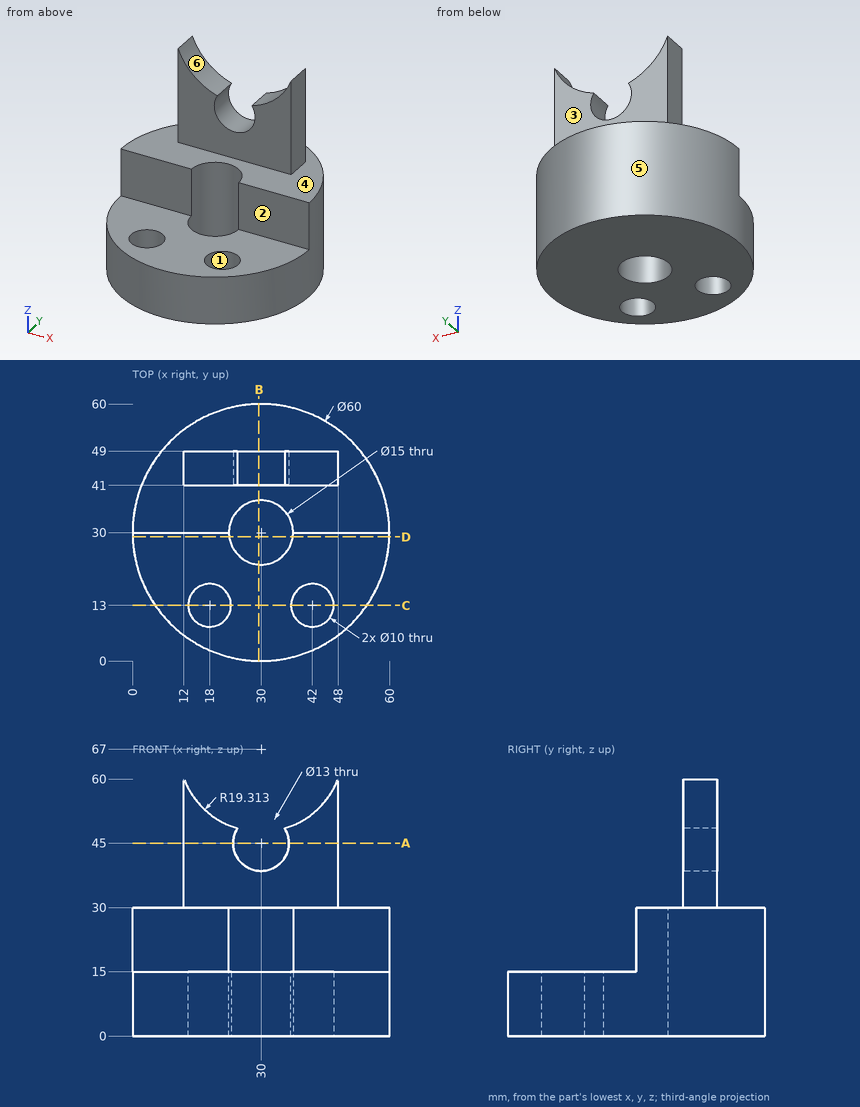
Source: three-view drawing plus pictorial views. Frame: mm from the lowest corner of the part. A direction names the side the tool comes from. Coordinates: 2 decimals unless noted, no trailing zeros. Order: outer loops, then holes, each group sorted by start corner. A loop starts at its lowest first (then second) coordinate and runs counter-clockwise, first axis right, second up. Notation, with made-up numbers: M -16.75,69 L 42.25,69 A14 ccw 42.25,84 Z; hole C -22,58.5 d11. An arc over 180 degrees is marked long. Write each question's results on one line, items separated by ' | '. Start each with the question number.
1. Section B-B, the plane x = 29.5. Return the cut outline in (y, z), then the cut area to 3 significant figures.
2. Section C-C, the plane y = 13. Return the cut outline in (x, z).
3. Reachability of the marked faces 1, 2 and 3 from +Z, -Z, +X, -X, +Y, -Y: full face, straight path, thin tool, end or side. Return the list, or none.
4. Pin query (flat end, axial travel): pin 1 (9 mm diameter, centred on x = 30, y = 30, fed in from -Z); pin 2 (1.5 mm diameter, centred on x = 26.5, y = 36.5, fed in from +Z); pin 3 (7.5 mm diameter, centred on x = 50.5, z = 24.5, fed in from -Y); pin 4 (10 mm diameter, centred on y = 36.5, z = 49, fed in from -X). Return the tip coordinate at first contact, or that it passes through.
5. Draft query along X for the marked faces 4, 5 and 6. Return one class per face: +X half, -X half, draft (parallel to the pull), parting line (faces both ways), or undercut.
6. Section D-D, the plane y = 29. Return the cut outline in (x, z).
7. Section A-A, the plane z = 45. Return the cut outline in (x, y), then the cut area to 3 significant figures.
8. Material intervals for L1, parallel to X at y = 44.75, z = 45; L2, parallel to Z at x = 57.5, y = 25.5; L3, parallel to Z at x = 30, y = 45, sorted ascending.
Solution:
1) outline: M 0,0 L 22.52,0 L 22.52,15 L 0,15 Z; M 37.48,0 L 60,0 L 60,30 L 49,30 L 49,38.52 L 41,38.52 L 41,30 L 37.48,30 Z | area: 1,080 mm²
2) outline: M 5.28,0 L 13,0 L 13,15 L 5.28,15 Z; M 23,0 L 37,0 L 37,15 L 23,15 Z; M 47,0 L 54.72,0 L 54.72,15 L 47,15 Z
3) face 1: +Z, -Z | face 2: +Z, +X, -X, -Y | face 3: +Z, +X, -X, +Y
4) pin 1: through | pin 2: z = 30 | pin 3: y = 30 | pin 4: x = 12
5) face 4: draft | face 5: parting line | face 6: undercut
6) outline: M 0.02,0 L 22.57,0 L 22.57,15 L 0.02,15 Z; M 37.43,0 L 59.98,0 L 59.98,15 L 37.43,15 Z
7) outline: M 12,41 L 23.5,41 L 23.5,49 L 12,49 Z; M 36.5,41 L 48,41 L 48,49 L 36.5,49 Z | area: 184 mm²
8) L1: 12 to 23.5, 36.5 to 48 | L2: 0 to 15 | L3: 0 to 38.5
